Autodesk Inventor part; units mm, degrees
ref_plane "YZ Plane" through (0, 0, 0) normal (1, 0, 0) x (0, 1, 0)
ref_plane "XZ Plane" through (0, 0, 0) normal (0, 1, 0) x (-1, 0, 0)
ref_plane "XY Plane" through (0, 0, 0) normal (0, 0, 1) x (1, 0, 0)
ref_plane "작업 평면1" through (0, 0, 0) normal (0, 0, 1) x (1, 0, 0)
sketch "스케치1" plane through (0, 0, 0) normal (0, 0, 1) x (1, 0, 0)
  arc A0 (-19.5808, 6.2636) -> (-20.1, 4.5766) centre (-17.1, 4.5766) ccw
  line L0 (-20.1, -39.6766) -> (-20.1, 4.5766)
  arc A1 (-20.1, -39.6766) -> (-19.5808, -41.3636) centre (-17.1, -39.6766) ccw
  line L1 (-15.8929, -46.7869) -> (-19.5808, -41.3636)
  arc A2 (-15.8929, -46.7869) -> (-13.4121, -48.1) centre (-13.4121, -45.1) ccw
  line L2 (13.4121, -48.1) -> (-13.4121, -48.1)
  arc A3 (13.4121, -48.1) -> (15.8929, -46.7869) centre (13.4121, -45.1) ccw
  line L3 (19.5808, -41.3636) -> (15.8929, -46.7869)
  arc A4 (19.5808, -41.3636) -> (20.1, -39.6766) centre (17.1, -39.6766) ccw
  line L4 (20.1, 4.5766) -> (20.1, -39.6766)
  arc A5 (20.1, 4.5766) -> (19.5808, 6.2636) centre (17.1, 4.5766) ccw
  line L5 (15.5953, 12.1246) -> (19.5808, 6.2636)
  arc A6 (15.5953, 12.1246) -> (13.9414, 13) centre (13.9414, 11) ccw
  line L6 (7.65, 13) -> (13.9414, 13)
  arc A7 (9.15, 11.5) -> (7.65, 13) centre (7.65, 11.5) ccw
  line L7 (9.15, 11.5) -> (9.15, 10)
  arc A8 (9.15, 10) -> (11.5, 7.65) centre (11.5, 10) ccw
  line L8 (11.5, 7.65) -> (13.5, 7.65)
  arc A9 (14.5, 6.65) -> (13.5, 7.65) centre (13.5, 6.65) ccw
  line L9 (14.5, 6.65) -> (14.5, -36.15)
  arc A10 (13.5, -37.15) -> (14.5, -36.15) centre (13.5, -36.15) ccw
  line L10 (13.5, -37.15) -> (11.5, -37.15)
  arc A11 (11.5, -37.15) -> (9.15, -39.5) centre (11.5, -39.5) ccw
  line L11 (9.15, -39.5) -> (9.15, -41.5)
  arc A12 (8.15, -42.5) -> (9.15, -41.5) centre (8.15, -41.5) ccw
  line L12 (8.15, -42.5) -> (-8.15, -42.5)
  arc A13 (-9.15, -41.5) -> (-8.15, -42.5) centre (-8.15, -41.5) ccw
  line L13 (-9.15, -41.5) -> (-9.15, -39.5)
  arc A14 (-9.15, -39.5) -> (-11.5, -37.15) centre (-11.5, -39.5) ccw
  line L14 (-11.5, -37.15) -> (-13.5, -37.15)
  arc A15 (-14.5, -36.15) -> (-13.5, -37.15) centre (-13.5, -36.15) ccw
  line L15 (-14.5, -36.15) -> (-14.5, 6.65)
  arc A16 (-13.5, 7.65) -> (-14.5, 6.65) centre (-13.5, 6.65) ccw
  line L16 (-13.5, 7.65) -> (-11.5, 7.65)
  arc A17 (-11.5, 7.65) -> (-9.15, 10) centre (-11.5, 10) ccw
  line L17 (-9.15, 10) -> (-9.15, 11.5)
  arc A18 (-7.65, 13) -> (-9.15, 11.5) centre (-7.65, 11.5) ccw
  line L18 (-13.9414, 13) -> (-7.65, 13)
  arc A19 (-13.9414, 13) -> (-15.5953, 12.1246) centre (-13.9414, 11) ccw
  line L19 (-19.5808, 6.2636) -> (-15.5953, 12.1246)
  circle A20 centre (17.3, 4) radius 1.35
  circle A21 centre (17.3, -18) radius 1.35
  circle A22 centre (11, -45.3) radius 1.35
  circle A23 centre (-17.3, 4) radius 1.35
  circle A24 centre (-17.3, -18) radius 1.35
  circle A25 centre (-11, -45.3) radius 1.35
  circle A26 centre (17.3, -40) radius 1.35
  circle A27 centre (-17.3, -40) radius 1.35
  line L20 (-11.5, 7.65) -> (11.5, 7.65)
  line L21 (11.5, 7.65) -> (11.5, 13)
  line L22 (11.5, 13) -> (-11.5, 13)
  line L23 (-11.5, 13) -> (-11.5, 7.65)
  point P0 (0, 0)
extrude "돌출1" add sketch "스케치1" along normal blind 6 contours L19 A19 L18 L23 L16 A16 L15 A15 L14 A14 L13 A13 L12 A12 L11 A11 L10 A10 L9 A9 L8 L21 L6 A6 L5 A5 L4 A4 L3 A3 L2 A2 L1 A1 L0 A0 | L18 A18 L17 A17 L23 | L22 A7 L7 A8 L20 A17 L17 A18 | L6 L21 A8 L7 A7
sketch "스케치2" plane through (-13.9414, 13, 0) normal (0, 1, 0) x (1, 0, 0)
  circle A0 centre (18.8828, -3) radius 1.35
  circle A1 centre (9, -3) radius 1.35
  point P0 (13.9414, 0)
extrude "돌출2" cut sketch "스케치2" against normal blind 6
properties part number "_inner" material "PMMA 플라스틱"
Work out the finished part from the listing and answer in its coordinate system (mm). A direction names the side the tool comes from. Coordinates: 2 decimals unless noted, no trailing zeros. Order: outer loops, then holes, each group sorted by start corner. A loop starts at its lowest first (then second) coordinate and runs counter-clockwise, first axis right, second up. Notation, with made-up numbers: (30.5, -8) - (52.5, -8) arc R33 ccw to (52.5, 25) - close; hole circle Ø11 at (45.5, 66). An arc over 180 degrees is marked (long way). Put each result on its own line as item: value. Start each with the question number.
1) For a pull along Z with two mould halves and no side action, classify faces 3 (the cylindrical face through (5.56, 10.36, 4.2)), 4 (the cylindrical face through (14.834, -47.742, 2.958)), 5 (the flat face through (15, -20, 6)) as released by +Z, released by -Z, zero draft, split by the parting line, or undercut.
2) A flat-ended cylindrical pin translates along its axis: pin 1 (1 mm diameter, centred on y = -40.5, z = 3.5, fed in from -X). Find the tip coordinate at first contact, or state that the pin passes through.
3) For faces 1 (the flat face through (0, -42.5, 3)), 2 (the flat face through (17.56, 9.235, 2.958)), determine the directions among +Z, -Z, +X, -X, +Y, -Y from which every point of the face is accessible in a straight line to the end or side of a thin tool.
4) Find the intervals of material crossed by line 1 (X direction, y = 10.65, z = 3); line 2 (X direction, y = -22, z = 5.25); line 3 (Y direction, x = -13, z = 1.2), in increasing order. Write a range as from..to.
5) Find section A-A (y = -18). Give the vertices of the cut face in (x, z).
6) Find section C-C (z = 3). State how many separate pieces and enclosed holes the cut face has, plus the area to 3 significant figures.
7) Find section B-B (y = -28). Give the vertices of the cut face in (x, z).
8) Find section D-D (x = -17.3). Give the vertices of the cut face in (y, z), plus the area to 3 significant figures.
Results list:
1. face 3: undercut
1. face 4: zero draft
1. face 5: released by +Z
2. pin 1: stops at x = -20.08
3. face 1: +Z, -Z
3. face 2: +Z, -Z, +X, +Y
4. line 1: x = -16.6..-6.29, -3.59..3.59, 6.29..16.6
4. line 2: x = -20.1..-14.5, 14.5..20.1
4. line 3: y = -48.1..-37.15, 7.65..13
5. outline: (-20.1, 0) - (-18.65, 0) - (-18.65, 6) - (-20.1, 6) - close; (-15.95, 0) - (-14.5, 0) - (-14.5, 6) - (-15.95, 6) - close; (14.5, 0) - (15.95, 0) - (15.95, 6) - (14.5, 6) - close; (18.65, 0) - (20.1, 0) - (20.1, 6) - (18.65, 6) - close
6. separate pieces: 2
6. enclosed holes: 8
6. area: 905 mm^2
7. outline: (-20.1, 0) - (-14.5, 0) - (-14.5, 6) - (-20.1, 6) - close; (14.5, 0) - (20.1, 0) - (20.1, 6) - (14.5, 6) - close
8. outline: (-44.72, 0) - (-41.35, 0) - (-41.35, 6) - (-44.72, 6) - close; (-38.65, 0) - (-19.35, 0) - (-19.35, 6) - (-38.65, 6) - close; (-16.65, 0) - (2.65, 0) - (2.65, 6) - (-16.65, 6) - close; (5.35, 0) - (9.62, 0) - (9.62, 6) - (5.35, 6) - close
8. area: 277 mm^2
